```python
from build123d import *

# Parameters (mm, degrees)
BOSS_EXTRUDE1_DEPTH = 5.5


with BuildPart() as part:
    # Sketch1 → Boss-Extrude1 (new body)
    with BuildSketch(Plane.XY):
        Polygon((16.666666667, 0), (33.333333333, 0), (33.333333333, -5.5), (50, -5.5), (50, 0), (50, 13.333333333), (55.5, 13.333333333), (55.5, 26.666666667), (50, 26.666666667), (50, 40), (33.333333333, 40), (33.333333333, 45.5), (16.666666667, 45.5), (16.666666667, 40), (0, 40), (-5.5, 40), (-5.5, 26.666666667), (0, 26.666666667), (0, 13.333333333), (-5.5, 13.333333333), (-5.5, -5.5), (0, -5.5), (16.666666667, -5.5), align=None)
    extrude(amount=BOSS_EXTRUDE1_DEPTH)


solid = part.part
```
Design review of the part built by this model. Coordinates are the model's own, in mm. A direction names the side the tool comes from. Coordinates: 2 decimals unless noted, no trailing zeros. Order: outer loops, then holes, each group sorted by start corner. A loop starts at its lowest first (then second) coordinate and runs counter-clockwise, first axis right, second up.
1) Take a section at B-B, the plane y = 24. Give the boundary of the cut face in (x, z), and give its area (3 significant figures).
2) For faces 5 (the flat face through (6, 40, 3)), 6 (the flat face through (-3, 26.667, 3)), 7 (the flat face through (53, 26.667, 3)), list the 3-axis set-ups (+Z, -Z, +X, -X, +Y, -Y) from which the entire face can be reached by the end or side of a thin tool; tool diameter is ignored.
3) Mouldability with a two-part tool opening along X and no side actions: class faces 1 (the flat face through (33.333, -3, 3)), 2 (the flat face through (50, 4, 3)), 3 (the flat face through (25, 20, 0)), 4 (the flat face through (-5.5, 4, 3)) as +X half, -X half, draft (parallel to the pull), parting line (faces both ways), or undercut.
4) Clearance check with flat-ended pins moving along their axes: pin 1 (1.6 mm diameter, centred on x = -2, z = 4, fed in from +Y); pin 2 (1.6 mm diameter, centred on y = 3.5, z = 4, fed in from +X); pin 3 (3 mm diameter, centred on x = 26, z = 3, fed in from -Y). State where each tip first meets the part, or that it passes through.
5) Wall thickness on line 1 along Y through (x, z) = (28, 4.5); line 2 along X through (y, z) = (33.5, 5.15); line 3 along Y through (x, z) = (53.5, 4.45): over which ranges is each line inside the solid? List them lowest first.
6) Take a section at A-A, the plane z = 1.6. Give the boundary of the cut face in (x, y), and give its area (3 significant figures).
7) Take a section at C-C, the plane x = 13. Give the boundary of the cut face in (y, z), and give its area (3 significant figures).
Returned:
1. outline: (0, 0) - (55.5, 0) - (55.5, 5.5) - (0, 5.5) - close
1. area: 305 mm2
2. face 5: +Z, -Z, -X, +Y
2. face 6: +Z, -Z, -X
2. face 7: +Z, -Z, +X, +Y
3. face 1: undercut
3. face 2: +X half
3. face 3: draft
3. face 4: -X half
4. pin 1: stops at y = 40
4. pin 2: stops at x = 50
4. pin 3: stops at y = 0
5. line 1: y = 0 to 45.5
5. line 2: x = -5.5 to 50
5. line 3: y = 13.33 to 26.67
6. outline: (-5.5, -5.5) - (16.67, -5.5) - (16.67, 0) - (33.33, 0) - (33.33, -5.5) - (50, -5.5) - (50, 13.33) - (55.5, 13.33) - (55.5, 26.67) - (50, 26.67) - (50, 40) - (33.33, 40) - (33.33, 45.5) - (16.67, 45.5) - (16.67, 40) - (-5.5, 40) - (-5.5, 26.67) - (0, 26.67) - (0, 13.33) - (-5.5, 13.33) - close
6. area: 2,530 mm2
7. outline: (-5.5, 0) - (40, 0) - (40, 5.5) - (-5.5, 5.5) - close
7. area: 250 mm2
